Verification items for the finished model (mm, model axes). Face numbers are marked on the shaded views. A direction names the side the tool comes from. Coordinates: 2 decimals unless noted, no trailing zeros. Loops run counter-clockwise (first coordinate to the right, second up) from the corner with the lowest first, then second, coordinate; pieces in that order, holes last.
Q1. Sectioned sample at C-C (z = 2). Enter the section's corners in (x, y), then the cut area to 3 significant figures.
Q2. Sectioned sample at B-B (x = -6). Enter the section's corners in (y, z).
Q3. Sectioned sample at A-A (z = 0). Enter the section's corners in (x, y), then the cut area to 3 significant figures.
Q4. Go/stop test with flat-tipped pins: P1, Ø0.9, axis at x = 8.5, z = 0, coming from the +Y side; P2, Ø4, axis at x = 8, z = 6.5, coming from the +Y side; P3, Ø1.5, axis at x = 1.5, z = 6.5, coming from the -Y side. Record where each tip stops, or that it passes through.
Q5. Material ranges on probe 1 along X at (y, z) = (15.6, 0); probe 2 along Y at (x, z) = (0, 0.5); probe 3 along X at (y, z) = (0, -1), recorded low to high.
Q6. Sectioned sample at D-D (x = -0.75). Enter the section's corners in (y, z).
Q7. Access from +Z, -Z, +X, -X, +Y, -Y to the whole of each face (thin tool, end or side, straight path). Record for the marked faces 1, 2 and 3.
```python
from build123d import *

# Parameters (mm, degrees)
LINK1_BODY_DEPTH       = 8.5
TONGUE_CUT_DEPTH       = 29.744564704
TONGUE_CUT_DEPTH_BACK  = 29.744564704
SKETCH1_W              = 5.5
SKETCH1_H              = 15.998130079
PIN_HOLES_DEPTH        = 26.64176281
PIN_HOLES_DEPTH_BACK   = 26.64176281
SKETCH3_R              = 1.1
SKETCH4_W              = 3.5
SKETCH4_H              = 2
GUIDE_BLOCK_1_DEPTH    = 2.5
CORD_GUIDES_DEPTH      = 27.673957337
CORD_GUIDES_DEPTH_BACK = 27.673957337
SKETCH6_R              = 0.6


with BuildPart() as part:
    # Link1_Outline → Link1_Body (new, symmetric)
    with BuildSketch(Plane.XY):
        with BuildLine():
            Line((-7.5, 0), (-7.5, 15.5))
            ThreePointArc((-7.5, 15.5), (0, 23), (7.5, 15.5))
            Line((7.5, 15.5), (7.5, 0))
            ThreePointArc((7.5, 0), (0, -7.5), (-7.5, 0))
        make_face()
    extrude(amount=LINK1_BODY_DEPTH, both=True)

    # Sketch1 → Tongue_Cut (cut, two sides: drawn at the far end of the back side and taken through both)
    with BuildSketch(Plane(origin=(7.5, 0, 0), x_dir=(0, 0, -1), z_dir=(1, 0, 0)).offset(-TONGUE_CUT_DEPTH_BACK)):
        with Locations((6.25, -0.00093496)):
            Rectangle(SKETCH1_W, SKETCH1_H)
        with Locations((-6.25, -0.00093496)):
            Rectangle(SKETCH1_W, SKETCH1_H)
    extrude(amount=TONGUE_CUT_DEPTH + TONGUE_CUT_DEPTH_BACK, mode=Mode.SUBTRACT)

    # Sketch3 → Pin_Holes (cut, two sides: drawn at the far end of the back side and taken through both)
    with BuildSketch(Plane.XY.offset(-PIN_HOLES_DEPTH_BACK)):
        Circle(SKETCH3_R)
    extrude(amount=PIN_HOLES_DEPTH + PIN_HOLES_DEPTH_BACK, mode=Mode.SUBTRACT)

    # Sketch4 → Guide_Block_1 (add, symmetric)
    with BuildSketch(Plane.XY):
        with Locations((8.75, 15)):
            Rectangle(SKETCH4_W, SKETCH4_H)
    extrude(amount=GUIDE_BLOCK_1_DEPTH, both=True)

    # Sketch6 → Cord_Guides (cut, two sides: drawn at the far end of the back side and taken through both)
    with BuildSketch(Plane(origin=(0, 0, 0), x_dir=(1, 0, 0), z_dir=(0, 1, 0)).offset(-CORD_GUIDES_DEPTH_BACK)):
        with Locations(Location((9, 0, 0), (0, 0, 90))):
            Circle(SKETCH6_R)
    extrude(amount=CORD_GUIDES_DEPTH + CORD_GUIDES_DEPTH_BACK, mode=Mode.SUBTRACT)


solid = part.part
```
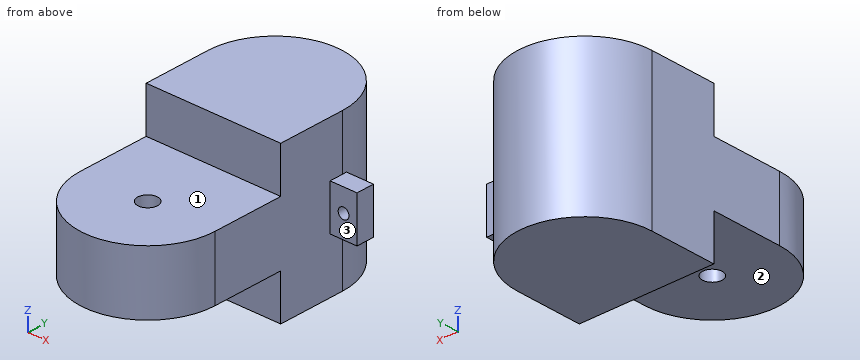
Geometry check:
1. outline: (-7.5, 0) arc R7.5 ccw to (7.5, 0) - (7.5, 14) - (10.5, 14) - (10.5, 16) - (7.48, 16) arc R7.5 ccw to (-7.5, 15.5) - close; hole circle Ø2.2 at (0, 0)
1. area: 411 mm2
2. outline: (-4.5, -3.5) - (8, -3.5) - (8, -8.5) - (20, -8.5) - (20, 8.5) - (8, 8.5) - (8, 3.5) - (-4.5, 3.5) - close
3. outline: (-7.5, 0) arc R7.5 ccw to (7.5, 0) - (7.5, 14) - (8.4, 14) - (8.4, 16) - (7.48, 16) arc R7.5 ccw to (-7.5, 15.5) - close; (9.6, 14) - (10.5, 14) - (10.5, 16) - (9.6, 16) - close; hole circle Ø2.2 at (0, 0)
3. area: 409 mm2
4. P1: stops at y = 16
4. P2: stops at y = 20
4. P3: stops at y = 8
5. probe 1: x = -7.5 to 8.4, 9.6 to 10.5
5. probe 2: y = -7.5 to -1.1, 1.1 to 23
5. probe 3: x = -7.5 to -1.1, 1.1 to 7.5
6. outline: (-7.46, -3.5) - (-0.8, -3.5) - (-0.8, 3.5) - (-7.46, 3.5) - close; (0.8, -3.5) - (8, -3.5) - (8, -8.5) - (22.96, -8.5) - (22.96, 8.5) - (8, 8.5) - (8, 3.5) - (0.8, 3.5) - close
7. face 1: +Z, +X, -X, -Y
7. face 2: -Z, +X, -X, -Y
7. face 3: +Z, -Z, +X, -Y
